Design review of the part shown in the three views and the two pictorial views. Dimensions are in mm from the part's minimum x, y and z. Coordinates: 2 decimals unless noted, no trailing zeros. Order: outer loops, then holes, each group sorted by start corner. A loop starts at its lowest first (then second) coordinate and runs counter-clockwise, first axis right, second up. Notation, with made-up numbers: M 27,44.25 L 50,44.25 A28 cw 50,75.25 Z; hole C 6,10 d6. An arc over 180 degrees is marked long. Use CSV: the item, a comma, the result in double quotes.
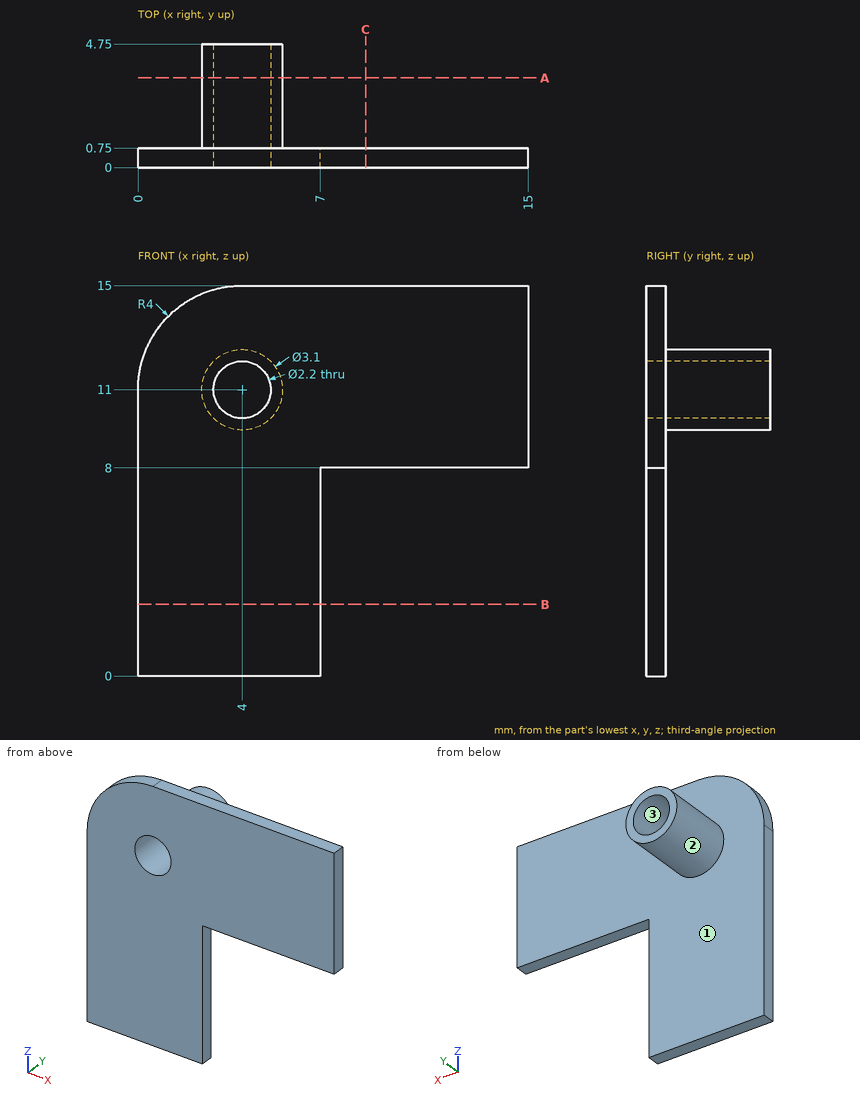
(1) The part is to be moulded in two halves that separate along Z. For the marked faces 1, 2 and 3, say which applies: pulls with the +Z half, pulls with the -Z half, needs draft (parallel to the pull), parting line crosses it, or undercut.
The answers:
face 1,"needs draft"
face 2,"parting line crosses it"
face 3,"undercut"
(2) Clearance check with flat-ended pins moving along their axes: P1, Ø0.6, axis at y = 0.5, z = 2.5, coming from the +X side; P2, Ø8, axis at x = 10, z = 10, coming from the +Y side; P3, Ø0.6, axis at x = 12, y = 0.5, coming from the -Z side. State where each tip first meets the part, or that it passes through.
The answers:
P1,"stops at x = 7"
P2,"stops at y = 0.75"
P3,"stops at z = 8"
(3) Add section A-A on y = 3.45. State the section outline as (x, z) points.
The answers:
outline,"C 4,11 d3.1; hole C 4,11 d2.2"
(4) Wall thickness on probe 1 along X at (y, z) = (3.2, 11); probe 2 along Z at (x, y) = (4, 2.3); probe 3 along Y at (x, z) = (12.25, 11.5): over which ranges is each line inside the solid? List them lowest first.
The answers:
probe 1,"x = 2.45 to 2.9, 5.1 to 5.55"
probe 2,"z = 9.45 to 9.9, 12.1 to 12.55"
probe 3,"y = 0 to 0.75"
(5) Add section B-B on z = 2.75. State the section outline as (x, y) points.
The answers:
outline,"M 0,0 L 7,0 L 7,0.75 L 0,0.75 Z"
(6) Add section C-C on x = 8.75. State the section outline as (y, z) points.
The answers:
outline,"M 0,8 L 0.75,8 L 0.75,15 L 0,15 Z"
